```python
from build123d import *

# Parameters (mm, degrees)
BOSS_EXTRUDE1_DEPTH            = 24
CUT_EXTRUDE1_DEPTH             = 25
SKETCH3_W                      = 7.55
SKETCH3_H                      = 24
F_4_5_4_5_DIAMETER_HOLE1_D     = 4.5
F_4_5_4_5_DIAMETER_HOLE1_DEPTH = 6
CHAMFER1_SIZE                  = 8
CUT_EXTRUDE2_DEPTH             = 21.045442769


with BuildPart() as part:
    # Sketch1 → Boss-Extrude1 (new body)
    with BuildSketch(Plane(origin=(0, 24, 0), x_dir=(1, 0, 0), z_dir=(0, 1, 0))):
        with BuildLine():
            Line((0, 0), (47, 0))
            Line((47, 0), (47, 6))
            Line((47, 6), (38.5, 6))
            ThreePointArc((38.5, 6), (35.307693119, 7.131854655), (33.541354656, 10.021831577))
            ThreePointArc((33.541354656, 10.021831577), (23.505747016, 20.045434485), (13.49594739, 9.996059012))
            ThreePointArc((13.49594739, 9.996059012), (11.698748894, 7.121907302), (8.5, 6))
            Line((8.5, 6), (0, 6))
            Line((0, 6), (0, 0))
        make_face()
    extrude(amount=-BOSS_EXTRUDE1_DEPTH)

    # Sketch2 → Cut-Extrude1 (cut, through all)
    with BuildSketch(Plane.XZ):
        with BuildLine():
            Line((24.018633311, 0), (23.018633311, 0))
            Line((23.018633311, 0), (23.018633311, -2.489295869))
            ThreePointArc((23.018633311, -2.489295869), (23.518633311, -2.472721384), (24.018633311, -2.489295869))
            Line((24.018633311, -2.489295869), (24.018633311, 0))
        make_face()
    extrude(amount=-CUT_EXTRUDE1_DEPTH, mode=Mode.SUBTRACT)

    # Sketch3 → Cut-Revolve1 (revolve, cut)
    with BuildSketch(Plane(origin=(0, 0, -10.022721384), x_dir=(-1, 0, 0), z_dir=(0, 0, -1))):
        with Locations((-27.293633311, 12)):
            Rectangle(SKETCH3_W, SKETCH3_H)
    revolve(axis=Axis((23.518633311, 0, -10.022721384), (0, 1, 0)), mode=Mode.SUBTRACT)

    # Ø4.5 (4.5) Diameter Hole1
    with Locations(Plane(origin=(0, 0, -6), x_dir=(-1, 0, 0), z_dir=(0, 0, -1))):
        with Locations((-41.037266621, 12), (-6, 12)):
            Hole(F_4_5_4_5_DIAMETER_HOLE1_D / 2, depth=F_4_5_4_5_DIAMETER_HOLE1_DEPTH)

    # Chamfer1
    chamfer1_edges = [part.edges().sort_by_distance(p)[0] for p in [
        (47, 0, -3),
        (0, 24, -3),
        (0, 0, -3),
        (47, 24, -3),
    ]]
    chamfer(chamfer1_edges, length=CHAMFER1_SIZE)

    # Sketch7 → Cut-Extrude2 (cut, through all)
    with BuildSketch(Plane.XY):
        with BuildLine():
            Line((41, 14.25), (43, 14.25))
            ThreePointArc((43, 14.25), (45.25, 12), (43, 9.75))
            Line((43, 9.75), (41, 9.75))
            ThreePointArc((41, 9.75), (38.75, 12), (41, 14.25))
        make_face()
        with BuildLine():
            Line((6, 9.75), (3.75, 9.75))
            ThreePointArc((3.75, 9.75), (1.5, 12), (3.75, 14.25))
            Line((3.75, 14.25), (6, 14.25))
            ThreePointArc((6, 14.25), (8.25, 12), (6, 9.75))
        make_face()
    extrude(amount=-CUT_EXTRUDE2_DEPTH, mode=Mode.SUBTRACT)


solid = part.part
```
CAD build for the part. Positions are in the model's coordinates, mm. A direction names the side the tool comes from. Round coordinates to 2 decimals unless told otherwise and drop trailing zeros. Order: outer loops, then holes, each group sorted by start corner. A loop starts at its lowest first (then second) coordinate and runs counter-clockwise, first axis right, second up. Notation, with made-up numbers: (40, 11) - (44, 11) arc R26 ccw to (44, 35) - close; hole circle Ø4 at (-39.75, -23.75). An arc over 180 degrees is marked (long way). Use CSV: the item, a comma, the result in double quotes. Start each with the question number.
1) Saw through at B-B (x = 43.5). List the corners of the cut face in (y, z).
2) Tool access for faces 1 (the flat face through (5.3, 9.5, -6)), 2 (the flat face through (47, 12, -3)), 3 (the cylindrical face through (8.25, 11.95, -2.96)), 4 (the flat face through (24.019, 12, -1)), 5 (the flat face through (33, 12, 0)): list every direction of +Z, -Z, +X, -X, +Y, -Y with a clear straight run to the whole face (end or side of a thin tool).
3) Saw through at D-D (y = 19). List the corners of the cut face in (x, z), and give its area (3 significant figures).
4) Pin check, flat tips, straight feed: pin 1 Ø1 at (x, z) = (42, -2.5) entering from +Y; pin 2 Ø4 at (y, z) = (21, -9.5) entering from +X; pin 3 Ø1 at (x, z) = (41.5, -3.5) entering from -Y. Stop position of each tip, or through.
5) Saw through at C-C (z = -5.5). List the corners of the cut face in (x, y), and give its area (3 significant figures).
6) Wall check: L1, parallel to X at y = 3.25, z = -10; L2, parallel to X at y = 11.5, z = -2; L3, parallel to Z at x = 45, y = 8. Give the ranges that are in metal, low to high. Write a range as [from, to].
7) Two-plate mould, pull along Y, no slides. Class faces 6 (the flat face through (41.9, 9.5, -6)), 7 (the cylindrical face through (38.75, 11.95, -2.96)), 8 (the flat face through (4, 20, -3)), 9 (the flat face through (5, 9.75, -3)): pulls with the +Y half, pulls with the -Y half, needs draft (parallel to the pull), parting line crosses it, or undercut.
8) Saw through at A-A (y = 12). List the corners of the cut face in (x, z).
Values follow:
1,outline,"(4.5, -6) - (9.81, -6) - (9.81, 0) - (4.5, 0) - close; (14.19, -6) - (19.5, -6) - (19.5, 0) - (14.19, 0) - close"
2,face 1,"-Z, -X, +Y, -Y"
2,face 2,"+Z, -Z, +X, +Y, -Y"
2,face 3,"+Z, -Z"
2,face 4,"+Z, +Y, -Y"
2,face 5,"+Z, +X, -X, +Y, -Y"
3,outline,"(3, -6) - (8.5, -6) arc R5.12 cw to (13.5, -10) arc R10.02 ccw to (33.54, -10.02) arc R5.07 cw to (38.5, -6) - (44, -6) - (44, 0) - (24.02, 0) - (24.02, -2.49) arc R7.55 cw (long way) to (23.02, -2.49) - (23.02, 0) - (3, 0) - close"
3,area,"313 mm2"
4,pin 1,"stops at y = 21.5"
4,pin 2,"stops at x = 34.9"
4,pin 3,"stops at y = 2"
5,outline,"(0, 8) - (8, 0) - (17.47, 0) - (17.47, 24) - (8, 24) - (0, 16) - close; (29.56, 0) - (39, 0) - (47, 8) - (47, 16) - (39, 24) - (29.56, 24) - close; hole (3.75, 9.75) - (6, 9.75) arc R2.25 ccw to (6, 14.25) - (3.75, 14.25) arc R2.25 ccw to start; hole (41, 9.75) - (43, 9.75) arc R2.25 ccw to (43, 14.25) - (41, 14.25) arc R2.25 ccw to start"
5,area,"659 mm2"
6,L1,"x = [13.5, 15.97], [31.07, 33.55]"
6,L2,"x = [0, 1.56], [8.19, 23.02], [24.02, 38.81], [45.19, 47]"
6,L3,"z = [-6, 0]"
7,face 6,"needs draft"
7,face 7,"undercut"
7,face 8,"pulls with the +Y half"
7,face 9,"undercut"
8,outline,"(0, -6) - (1.5, -6) - (1.5, 0) - (0, 0) - close; (8.25, -6) - (8.5, -6) arc R5.12 cw to (13.5, -10) arc R10.02 ccw to (33.54, -10.02) arc R5.07 cw to (38.5, -6) - (38.75, -6) - (38.75, 0) - (24.02, 0) - (24.02, -2.49) arc R7.55 cw (long way) to (23.02, -2.49) - (23.02, 0) - (8.25, 0) - close; (45.25, -6) - (47, -6) - (47, 0) - (45.25, 0) - close"
